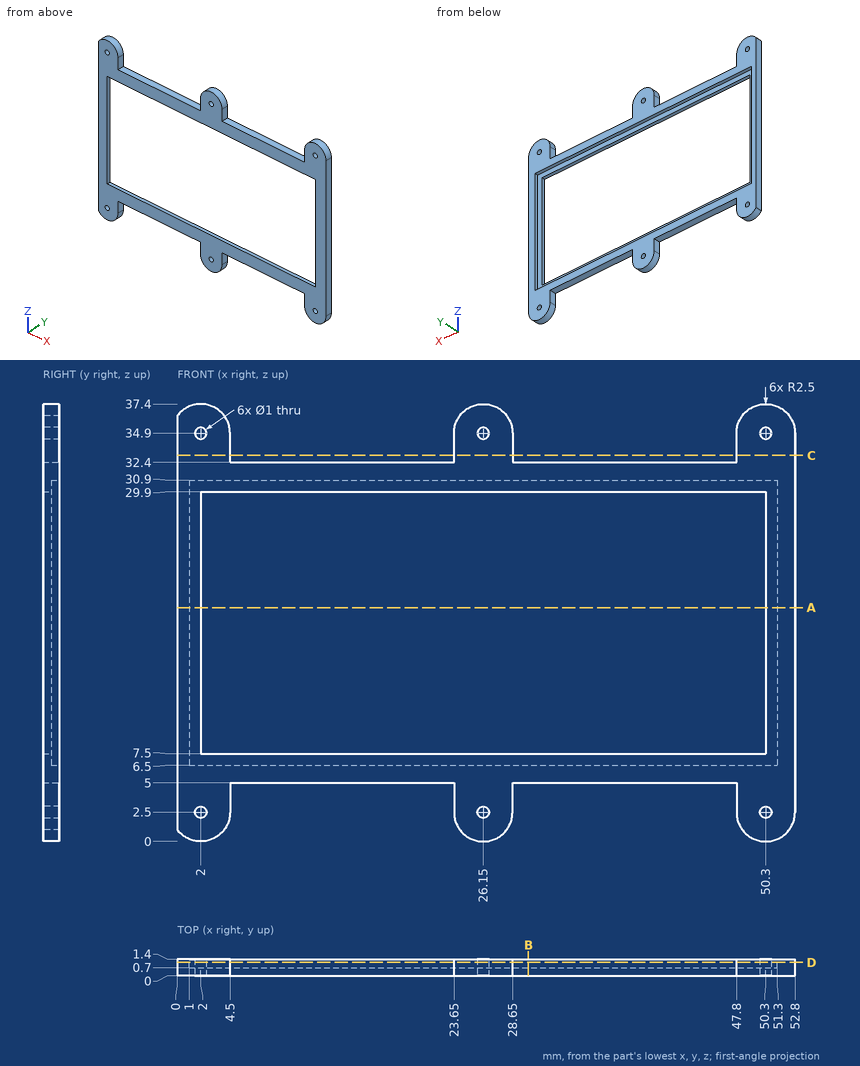
Answer from the drawing. Dimensions are ordinates in mm from the lowest x, y and z of the part. Round coordinates to 2 decimals unless told otherwise and drop trailing zeros. Order: outer loops, then holes, each group sorted by start corner. A loop starts at its lowest first (then second) coordinate and runs counter-clockwise, first axis right, second up.
1) Straight lines are drawn through the part: L1, parallel to X at y = 0.8, z = 2.5; L2, parallel to Z at x = 2, y = 1; L3, parallel to Z at x = 26.15, y = 0.3. For each, find the intervals that lie inside material, in ascending order.
2) Flat-ended cylindrical pins translate along their axes: pin 1 (12 mm diameter, centred on x = 19, z = 33.5, fed in from +Y); pin 2 (0.7 mm diameter, centred on x = 12, y = 0.5, fed in from +Z). Find the tip coordinate at first contact, or state that the pin passes through.
3) The part is cut by section C-C on z = 33. Write down the section's boundary in (x, y), plus the area to 3 significant figures.
4) The part is cut by section D-D on y = 1.15. Give the number of separate pieces and of enclosed holes in the cut face, plus the area to 3 significant figures.
5) The part is cut by section B-B on x = 30. Write down the section's boundary in (y, z).
6) The part is cut by section A-A on z = 20. Write down the section's boundary in (x, y), plus the area to 3 significant figures.
Resolved:
1. L1: x = 0 to 1.5, 2.5 to 4.5, 23.65 to 25.65, 26.65 to 28.65, 47.8 to 49.8, 50.8 to 52.8
1. L2: z = 0 to 2, 3 to 6.5, 30.9 to 34.4, 35.4 to 37.4
1. L3: z = 0 to 2, 3 to 7.5, 29.9 to 34.4, 35.4 to 37.4
2. pin 1: stops at y = 1.4
2. pin 2: stops at z = 32.4
3. outline: (0, 0) - (4.5, 0) - (4.5, 1.4) - (0, 1.4) - close; (23.65, 0) - (28.65, 0) - (28.65, 1.4) - (23.65, 1.4) - close; (47.8, 0) - (52.8, 0) - (52.8, 1.4) - (47.8, 1.4) - close
3. area: 20.3 mm2
4. separate pieces: 1
4. enclosed holes: 7
4. area: 345 mm2
5. outline: (0, 5) - (1.4, 5) - (1.4, 6.5) - (0.7, 6.5) - (0.7, 7.5) - (0, 7.5) - close; (0, 29.9) - (0.7, 29.9) - (0.7, 30.9) - (1.4, 30.9) - (1.4, 32.4) - (0, 32.4) - close
6. outline: (0, 0) - (2, 0) - (2, 0.7) - (1, 0.7) - (1, 1.4) - (0, 1.4) - close; (50.3, 0) - (52.8, 0) - (52.8, 1.4) - (51.3, 1.4) - (51.3, 0.7) - (50.3, 0.7) - close
6. area: 4.90 mm2
